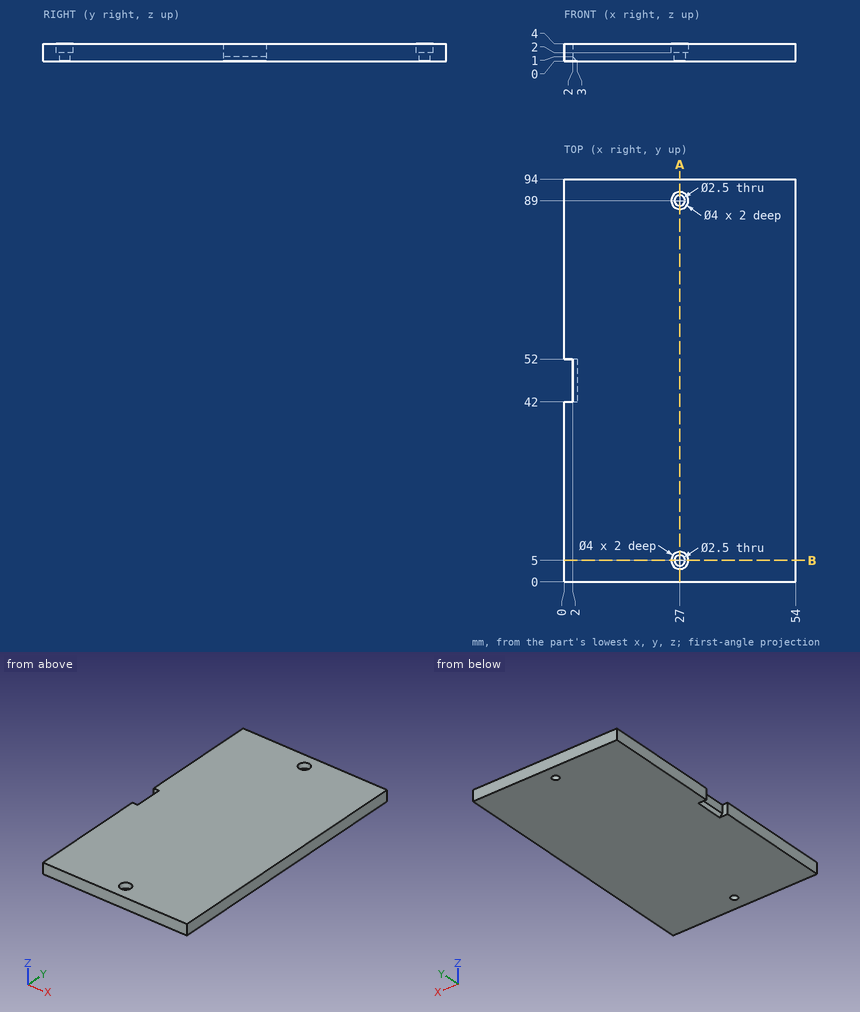
Geometry: see drawing. Coordinates: mm, zero at the bounding-box minimum. Give positions to 0.01 mm unless a question says otherwise; leave off trailing zeros. Loops run counter-clockwise (first coordinate to the right, second up) from the corner with the lowest first, then second, coordinate; pieces in that order, holes last. Notation, with made-up numbers: (69, -23) - (83, -23) arc R9 cw to (83, -12) - close; hole circle Ø7 at (32.5, 70.5). An arc over 180 degrees is marked (long way). Use CSV: the item, a comma, the result in double quotes.
1) Pin query (flat end, axial travel): P1, Ø3, axis at x = 27, y = 5, coming from the -Z side; P2, Ø0.9, axis at y = 47, z = 2, coming from the -X side; P3, Ø1.2, axis at x = 27.5, y = 4.5, coming from the +Z side. Return the tip coordinate at first contact, or that it passes through.
Worked out:
P1,"stops at z = 0"
P2,"stops at x = 2"
P3,"stops at z = 2"
2) Line query: line 1 (Y direction, x = 27, z = 1.1); line 2 (Y direction, x = 27, z = 2.4); line 3 (X direction, y = 89, z = 0.5). Output: solid intervals per line, ascending.
Worked out:
line 1,"y = 0 to 3.75, 6.25 to 87.75, 90.25 to 94"
line 2,"y = 0 to 3, 7 to 87, 91 to 94"
line 3,"x = 0 to 25.75, 28.25 to 54"
3) Cut plane B-B (y = 5). Output: boundary loops of the cut face in (x, z), and give its area (3 significant figures).
Worked out:
outline,"(0, 0) - (25.75, 0) - (25.75, 2) - (25, 2) - (25, 4) - (0, 4) - close; (28.25, 0) - (54, 0) - (54, 4) - (29, 4) - (29, 2) - (28.25, 2) - close"
area,"203 mm^2"
4) Cut plane A-A (x = 27). Output: boundary loops of the cut face in (y, z), and give its area (3 significant figures).
Worked out:
outline,"(0, 0) - (3.75, 0) - (3.75, 2) - (3, 2) - (3, 4) - (0, 4) - close; (6.25, 0) - (87.75, 0) - (87.75, 2) - (87, 2) - (87, 4) - (7, 4) - (7, 2) - (6.25, 2) - close; (90.25, 0) - (94, 0) - (94, 4) - (91, 4) - (91, 2) - (90.25, 2) - close"
area,"350 mm^2"
